Can you work these out from the model? Positions are in its coordinate system, mm. A direction names the side the tool comes from. Give positions to 0.01 mm unless a question says otherwise; leave off trailing zeros. Order: outer loops, then holes, each group sorted by start corner. A loop starts at its lowest first (then second) coordinate and runs counter-clockwise, first axis right, second up. Notation, with made-up numbers: (-4.75, 38.5) - (53.25, 38.5) arc R12 ccw to (53.25, 47.5) - close; hole circle Ø4 at (34.5, -9). An arc over 180 degrees is marked (long way). Use one line per item in the form item = value. Start each with the question number.
1) Suppose I cut it at A-A, the plane y = -1. Write out the boundary of the cut face in (x, z).
2) Please list where these lines run through material, in increasing order: probe 1 along Y at (x, z) = (-4.25, 4.4); probe 2 along Y at (x, z) = (7.75, 1.05); probe 3 along X at (y, z) = (-17, 3.4).
3) For pin 1 (0.9 mm diameter, centred on x = 8, z = 1.5, fed in from -Y); pin 2 (1.5 mm diameter, centred on y = 10, z = 0.5, fed in from +X); pin 3 (2.5 mm diameter, centred on x = -7.5, z = 3, fed in from +Y), each with a flat end and sliding along its axis, tell me the tip position at first contact or that it passes through.
4) Suppose I cut it at B-B, the plane y = 23. Write out the boundary of the cut face in (x, z), and give its area (3 significant figures).
5) Which directions (+Z, -Z, +X, -X, +Y, -Y) give clear straight access to the entire face, cutting with the end or side of a thin tool? Please do faces 4 (the flat face through (-8, 25, 2)), 5 (the flat face through (8, 0, 2)), 6 (the cylindrical face through (-6.113, 42.775, 2.465)).
6) We'd pull the mould along X, two halves only. Please class faces 1 (the cylindrical face through (-3.641, 1.203, 2.465)), 2 (the cylindrical face through (6.285, 42.804, 2.465)), 3 (the flat face through (-8, 0, 2)): released by +X, released by -X, zero draft, split by the parting line, or undercut.
```python
from build123d import *

# Parameters (mm, degrees)
F1_DEPTH = 5


with BuildPart() as f1:
    # F0 (on Top) → F1 (new body)
    with BuildSketch(Plane.XY):
        with BuildLine():
            Line((-6.658514, -11.222553), (-9.659046, -15.71237))
            ThreePointArc((-9.659046, -15.71237), (-9.953746, -16.27401), (-10.123783, -16.885054))
            ThreePointArc((-10.123783, -16.885054), (-10.334123, -18.760982), (-10.341643, -20.64865))
            Line((-10.341643, -20.64865), (-7.164773, -20.64865))
            ThreePointArc((-7.164773, -20.64865), (-3.5, -21.75704), (-7.164773, -22.865431))
            Line((-7.164773, -22.865431), (-10.088952, -22.865431))
            ThreePointArc((-10.088952, -22.865431), (-7.140782, -29.906834), (-1.480678, -35.028971))
            ThreePointArc((-1.480678, -35.028971), (0, -35.419834), (1.480678, -35.028971))
            ThreePointArc((1.480678, -35.028971), (8.658585, -27.317676), (10.123783, -16.885054))
            ThreePointArc((10.123783, -16.885054), (9.953746, -16.27401), (9.659046, -15.71237))
            Line((9.659046, -15.71237), (6.658514, -11.222553))
            ThreePointArc((6.658514, -11.222553), (6.456449, -7.114558), (9.984211, -5))
            Line((9.984211, -5), (9.496351, -5))
            ThreePointArc((9.496351, -5), (10.910565, -4.414214), (11.496351, -3))
            Line((11.496351, -3), (11.496351, -2))
            ThreePointArc((11.496351, -2), (10.910565, -0.585786), (9.496351, 0))
            Line((9.496351, 0), (6.5, 0))
            ThreePointArc((6.5, 0), (3.671573, 1.171573), (2.5, 4))
            Line((2.5, 4), (2.5, 6))
            ThreePointArc((2.5, 6), (3.671573, 8.828427), (6.5, 10))
            Line((6.5, 10), (9.496351, 10))
            ThreePointArc((9.496351, 10), (10.910565, 10.585786), (11.496351, 12))
            Line((11.496351, 12), (11.496351, 13))
            ThreePointArc((11.496351, 13), (10.910565, 14.414214), (9.496351, 15))
            Line((9.496351, 15), (6.5, 15))
            ThreePointArc((6.5, 15), (3.671573, 16.171573), (2.5, 19))
            Line((2.5, 19), (2.5, 21))
            ThreePointArc((2.5, 21), (3.671573, 23.828427), (6.5, 25))
            Line((6.5, 25), (9.496351, 25))
            ThreePointArc((9.496351, 25), (10.910565, 25.585786), (11.496351, 27))
            Line((11.496351, 27), (11.496351, 28))
            ThreePointArc((11.496351, 28), (10.910565, 29.414214), (9.496351, 30))
            Line((9.496351, 30), (6.5, 30))
            ThreePointArc((6.5, 30), (3.671573, 31.171573), (2.5, 34))
            Line((2.5, 34), (2.5, 37))
            Line((2.5, 37), (13, 42.171836))
            ThreePointArc((13, 42.171836), (13.498078, 43.410256), (12.321401, 44.040492))
            ThreePointArc((12.321401, 44.040492), (6.198921, 42.789454), (0, 42))
            ThreePointArc((0, 42), (-6.198921, 42.789454), (-12.321401, 44.040492))
            ThreePointArc((-12.321401, 44.040492), (-13.498078, 43.410256), (-13, 42.171836))
            Line((-13, 42.171836), (-2.5, 37))
            Line((-2.5, 37), (-2.5, 34))
            ThreePointArc((-2.5, 34), (-3.671573, 31.171573), (-6.5, 30))
            Line((-6.5, 30), (-9.496351, 30))
            ThreePointArc((-9.496351, 30), (-10.910565, 29.414214), (-11.496351, 28))
            Line((-11.496351, 28), (-11.496351, 27))
            ThreePointArc((-11.496351, 27), (-10.910565, 25.585786), (-9.496351, 25))
            Line((-9.496351, 25), (-6.5, 25))
            ThreePointArc((-6.5, 25), (-3.671573, 23.828427), (-2.5, 21))
            Line((-2.5, 21), (-2.5, 19))
            ThreePointArc((-2.5, 19), (-3.671573, 16.171573), (-6.5, 15))
            Line((-6.5, 15), (-9.496351, 15))
            ThreePointArc((-9.496351, 15), (-10.910565, 14.414214), (-11.496351, 13))
            Line((-11.496351, 13), (-11.496351, 12))
            ThreePointArc((-11.496351, 12), (-10.910565, 10.585786), (-9.496351, 10))
            Line((-9.496351, 10), (-6.5, 10))
            ThreePointArc((-6.5, 10), (-3.671573, 8.828427), (-2.5, 6))
            Line((-2.5, 6), (-2.5, 4))
            ThreePointArc((-2.5, 4), (-3.671573, 1.171573), (-6.5, 0))
            Line((-6.5, 0), (-9.496351, 0))
            ThreePointArc((-9.496351, 0), (-10.910565, -0.585786), (-11.496351, -2))
            Line((-11.496351, -2), (-11.496351, -3))
            ThreePointArc((-11.496351, -3), (-10.910565, -4.414214), (-9.496351, -5))
            Line((-9.496351, -5), (-9.984211, -5))
            ThreePointArc((-9.984211, -5), (-6.456449, -7.114558), (-6.658514, -11.222553))
        make_face()
    extrude(amount=F1_DEPTH)


solid = f1.part
```
Result sheet:
q1.outline = (-11.23, 0) - (11.23, 0) - (11.23, 5) - (-11.23, 5) - close
q2.probe_1 = -33.08 to -23.32, -20.2 to 0.69, 9.31 to 15.69, 24.31 to 30.69, 37.86 to 42.49
q2.probe_2 = -28.99 to -12.86, -5.68 to 0, 10 to 15, 25 to 30, 39.59 to 43.06
q2.probe_3 = -10.14 to 10.14
q3.pin_1 = -29.3
q3.pin_2 = 11.06
q3.pin_3 = 43.25
q4.outline = (-3.04, 0) - (3.04, 0) - (3.04, 5) - (-3.04, 5) - close
q4.area = 30.4 mm²
q5.face_4 = +Z, -Z, -X
q5.face_5 = +Z, -Z, +X
q5.face_6 = +Z, -Z, +Y
q6.face_1 = released by -X
q6.face_2 = undercut
q6.face_3 = zero draft
